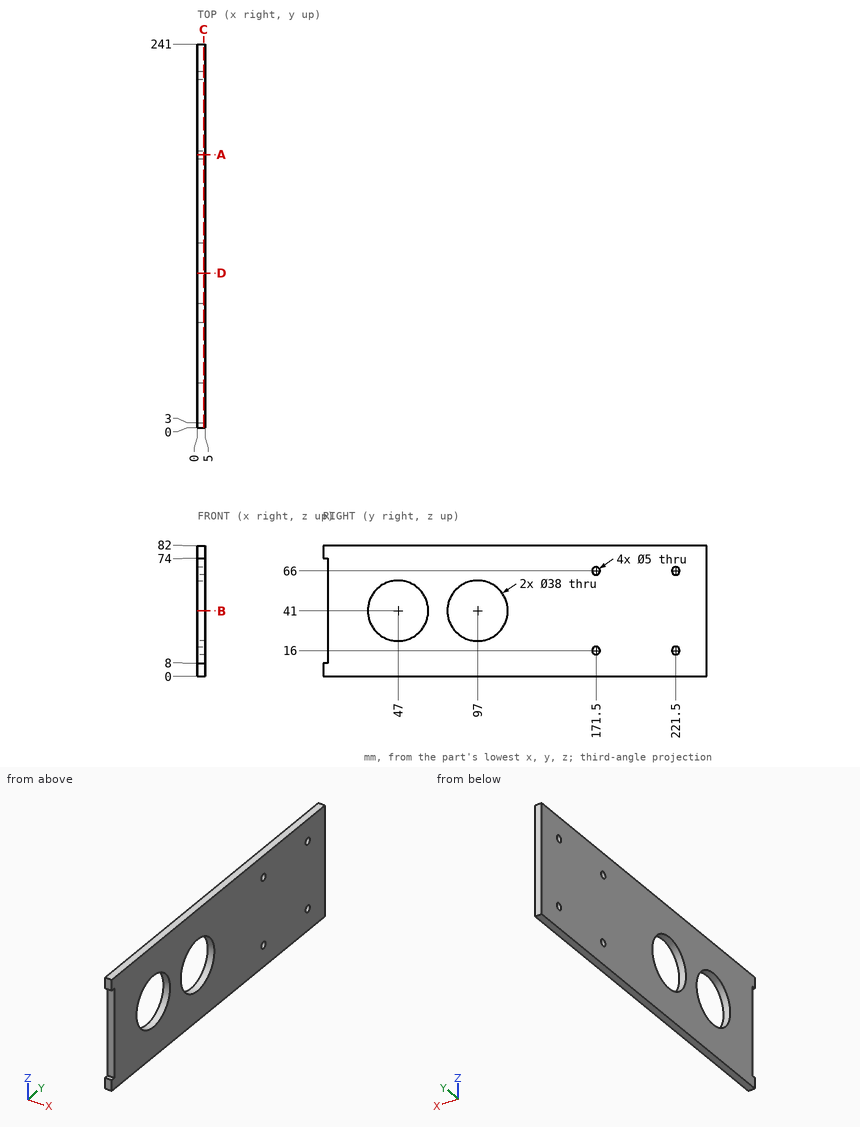
Print and shaded views of the part. All mm, measured from the part's lowest x, y and z. Coordinates: 2 decimals unless noted, no trailing zeros. Write each loop counter-clockwise with the first axis right and the second up, starting at its lowest first coordinate (ties: lowest second). Pieces come first, ordered by that corner, then holes. Notation, with made-up numbers: M 87.25,59.5 L 109.25,59.5 A20 ccw 109.25,94.5 Z; hole C 68,73 d11. An arc over 180 degrees is marked long. Return JSON: item names as keys, results as strings.
1. Saw through at C-C, the plane x = 4.05. Write the cut outline in (y, z), then the cut area to 3 significant figures.
Determined:
{"outline": "M 0,0 L 241,0 L 241,82 L 0,82 L 0,74 L 3,74 L 3,8 L 0,8 Z; hole C 47,41 d38; hole C 97,41 d38; hole C 171.5,16 d5; hole C 171.5,66 d5; hole C 221.5,16 d5; hole C 221.5,66 d5", "area": "17,200 mm²"}
2. Saw through at A-A, the plane y = 171.5. Write the cut outline in (x, z).
Determined:
{"outline": "M 0,0 L 5,0 L 5,13.5 L 0,13.5 Z; M 0,18.5 L 5,18.5 L 5,63.5 L 0,63.5 Z; M 0,68.5 L 5,68.5 L 5,82 L 0,82 Z"}
3. Saw through at B-B, the plane z = 41. Write the cut outline in (x, y), then the cut area to 3 significant figures.
Determined:
{"outline": "M 0,3 L 5,3 L 5,28 L 0,28 Z; M 0,66 L 5,66 L 5,78 L 0,78 Z; M 0,116 L 5,116 L 5,241 L 0,241 Z", "area": "810 mm²"}
4. Probe L1, parallel to Z at x = 1.65, y = 171.5; L2, parallel to Y at x = 1.25, z = 41; L3, parallel to Y at x = 3.1, z = 16. List the from-to ranges inside material, lowest first.
Determined:
{"L1": "0 to 13.5, 18.5 to 63.5, 68.5 to 82", "L2": "3 to 28, 66 to 78, 116 to 241", "L3": "3 to 169, 174 to 219, 224 to 241"}
5. Flat gauge pin, fed straight in: pin 1 Ø1 at (x, z) = (1, 27.5) entering from -Y. Where does the tip first touch, or does it go through?
Determined:
{"pin 1": "y = 3"}
6. Saw through at D-D, the plane y = 97. Write the cut outline in (x, z), then the cut area to 3 significant figures.
Determined:
{"outline": "M 0,0 L 5,0 L 5,22 L 0,22 Z; M 0,60 L 5,60 L 5,82 L 0,82 Z", "area": "220 mm²"}
